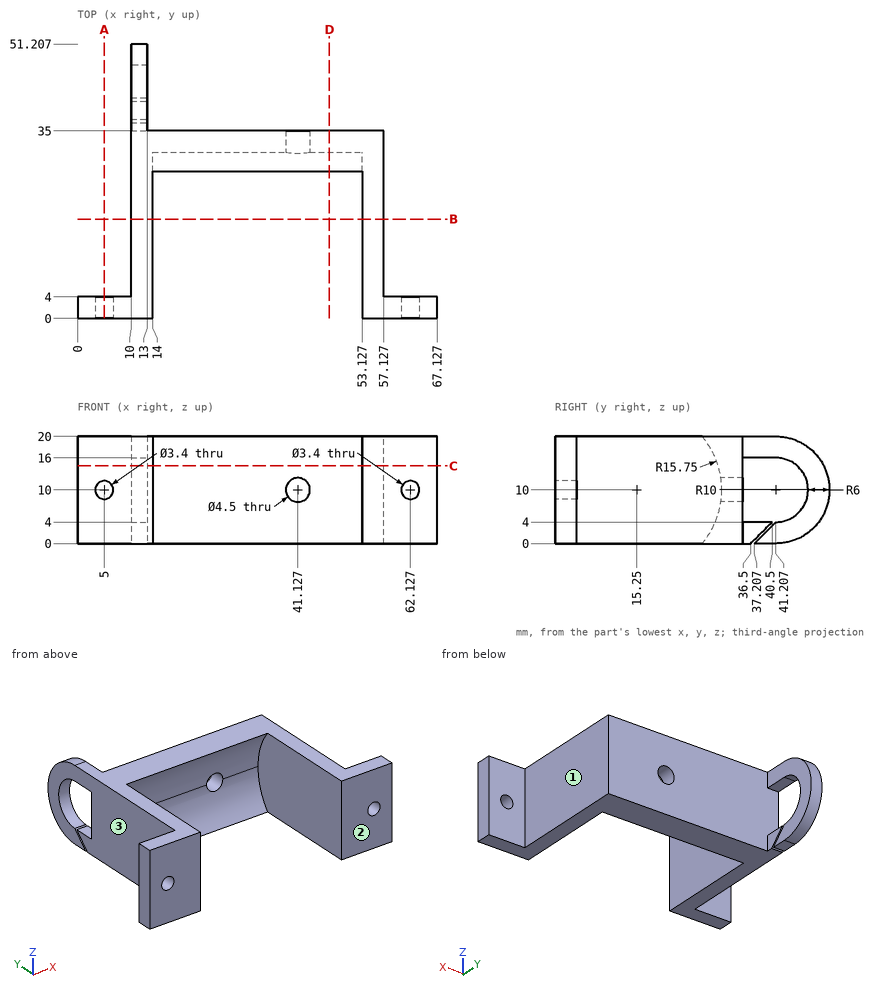
Here's the drawing with two shaded views (mm, measured from the low corner). I have some questions. A direction names the side the tool comes from. Coordinates: 2 decimals unless noted, no trailing zeros. Order: outer loops, then holes, each group sorted by start corner. A loop starts at its lowest first (then second) coordinate and runs counter-clockwise, first axis right, second up.
Q1. Which directions (+Z, -Z, +X, -X, +Y, -Y) give clear straight access to the entire face, cutting with the end or side of a thin tool? Please do the marked faces 1, 2 and 3.
Q2. Suppose I cut it at A-A on x = 5. Please give me the cut outline in (y, z), and give its area (3 significant figures).
Q3. Please list where these lines run through material, in increasing order: L1, parallel to X at y = 10.5, z = 9; L2, parallel to Z at x = 5, y = 2; L3, parallel to Y at x = 4, z = 14.
Q4. Suppose I cut it at C-C on z = 14.5. Please give me the cut outline in (x, y).
Q5. Suppose I cut it at D-D on x = 47. Please give me the cut outline in (y, z), and give its area (3 significant figures).
Q6. Will these pins go through, and if not, where does the flat tip stop? pin 1 (7 mm diameter, centred on x = 41.127, z = 10, fed in from +Y); pin 2 (8 mm diameter, centred on y = 30, z = 11.5, fed in from -X); pin 3 (1.5 mm diameter, centred on y = 23.5, z = 13.5, fed in from +X).
Q7. Suppose I cut it at B-B on y = 18.5. Please give me the cut outline in (x, z), and give its area (3 significant figures).
Answer:
1. face 1: +Z, -Z, +X, +Y
1. face 2: +Z, -Z, +X, -X, -Y
1. face 3: +Z, -Z, -X, +Y
2. outline: (0, 0) - (4, 0) - (4, 8.3) - (0, 8.3) - close; (0, 11.7) - (4, 11.7) - (4, 20) - (0, 20) - close
2. area: 66.4 mm2
3. L1: x = 10 to 14, 53.13 to 57.13
3. L2: z = 0 to 8.3, 11.7 to 20
3. L3: y = 0 to 4
4. outline: (0, 0) - (14, 0) - (14, 30.34) - (53.13, 30.34) - (53.13, 0) - (67.13, 0) - (67.13, 4) - (57.13, 4) - (57.13, 35) - (10, 35) - (10, 4) - (0, 4) - close; (10, 45.18) - (13, 45.18) - (13, 50.14) - (10, 50.14) - close
5. outline: (27.42, 0) - (35, 0) - (35, 20) - (27.42, 20) arc R15.75 cw to start
5. area: 103 mm2
6. pin 1: stops at y = 35
6. pin 2: stops at x = 10
6. pin 3: stops at x = 57.13
7. outline: (10, 0) - (14, 0) - (14, 20) - (10, 20) - close; (53.13, 0) - (57.13, 0) - (57.13, 20) - (53.13, 20) - close
7. area: 160 mm2
